Check sheet for the modelled part. Datum: model origin and axes. Units: mm. A direction names the side the tool comes from. Coordinates: 2 decimals unless noted, no trailing zeros. Write each loop counter-clockwise with the first axis right and the second up, starting at its lowest first coordinate (ties: lowest second). Pieces come first, ordered by that corner, then holes. Notation, with made-up numbers: M -25.75,-21 L 8.25,-21 A24 ccw 8.25,1 Z; hole C 26,6.5 d4. An arc over 180 degrees is marked long. Answer as CSV lines item,"result". Start each with the question number.
Q1. Sectioned sample at D-D, the plane z = -7. Record the cut outline in (x, y).
Q2. Sectioned sample at A-A, the plane x = 8. Record the cut outline in (y, z).
Q3. Sectioned sample at B-B, the plane z = -50. Record the cut outline in (x, y), then the cut area to 3 significant figures.
Q4. Sectioned sample at C-C, the plane y = 24. Record the cut outline in (x, z).
Q5. Thickness scan on line 1 along Y through (x, z) = (93, -72.5); line 2 along Z through (x, y) = (-72.5, -3); line 3 along Z through (x, y) = (-60, 14.5). Record the ranges inside material, lowest first. Write a range as from..to.
Q6. Depth check by flat-ended pin: pin 1 Ø16.5 at (x, y) = (285, -3.5) entering from -Z; pin 2 Ø16.5 at (y, z) = (-9.5, -47) entering from +X; pin 3 Ø22 at (x, y) = (50.5, 21.5) entering from -Z. Enter the tip coordinate at first touch or a pass-through.
Q7. Access from +Z, -Z, +X, -X, +Y, -Y to the whole of each face (thin tool, end or side, straight path). Record for faces 1 (the flat face through (13, 12.5, -63)), 2 (the flat face through (255, -7, -43)), 3 (the flat face through (-265, -7, -17.5)).
from build123d import *

# Parameters (mm, degrees)
SKETCH053_W     = 610
SKETCH053_H     = 165
PAD005_DEPTH    = 65
SKETCH054_W     = 60
SKETCH054_H     = 32
SKETCH054_W_2   = 70
SKETCH054_H_2   = 18
POCKET047_DEPTH = 165.001
SKETCH055_W     = 80
SKETCH055_H     = 32
SKETCH055_W_2   = 90
SKETCH055_H_2   = 18
POCKET048_DEPTH = 165.001
SKETCH056_W     = 50
SKETCH056_H     = 65
POCKET049_DEPTH = 65.001
SKETCH057_W     = 65
SKETCH057_H     = 65
POCKET050_DEPTH = 65.001
SKETCH059_W     = 610
SKETCH059_H     = 32
POCKET052_DEPTH = 10
SKETCH060_W     = 20
SKETCH060_H     = 25
POCKET053_DEPTH = 610.001
SKETCH061_W     = 50
SKETCH061_H     = 15
POCKET054_DEPTH = 610.001
SKETCH062_W     = 15
SKETCH062_H     = 65
POCKET055_DEPTH = 165.001
SKETCH063_W     = 10
SKETCH063_H     = 32.5
POCKET056_DEPTH = 165.001


with BuildPart() as part:
    # Sketch053 (on DatumPlane) → Pad005 (new body)
    with BuildSketch(Plane.XZ.offset(32.5)):
        Rectangle(SKETCH053_W, SKETCH053_H)
    extrude(amount=-PAD005_DEPTH)

    # Sketch054 (on DatumPlane) → Pocket047 (cut, through all)
    with BuildSketch(Plane.XY.offset(82.5)):
        with Locations((275, 16.5)):
            Rectangle(SKETCH054_W, SKETCH054_H)
        with Locations((270, -23.5)):
            Rectangle(SKETCH054_W_2, SKETCH054_H_2)
    extrude(amount=-POCKET047_DEPTH, mode=Mode.SUBTRACT)

    # Sketch055 (on DatumPlane) → Pocket048 (cut, through all)
    with BuildSketch(Plane.XY.offset(82.5)):
        with Locations((-265, 16.5)):
            Rectangle(SKETCH055_W, SKETCH055_H)
        with Locations((-260, -23.5)):
            Rectangle(SKETCH055_W_2, SKETCH055_H_2)
    extrude(amount=-POCKET048_DEPTH, mode=Mode.SUBTRACT)

    # Sketch056 (on DatumPlane) → Pocket049 (cut, through all)
    with BuildSketch(Plane.XZ.offset(32.5)):
        with Locations((280, -50)):
            Rectangle(SKETCH056_W, SKETCH056_H)
    extrude(amount=-POCKET049_DEPTH, mode=Mode.SUBTRACT)

    # Sketch057 (on DatumPlane) → Pocket050 (cut, through all)
    with BuildSketch(Plane.XZ.offset(32.5)):
        with Locations((-272.5, -50)):
            Rectangle(SKETCH057_W, SKETCH057_H)
    extrude(amount=-POCKET050_DEPTH, mode=Mode.SUBTRACT)

    # Sketch059 (on DatumPlane) → Pocket052 (cut)
    with BuildSketch(Plane.XY.offset(82.5)):
        with Locations((0, 16.5)):
            Rectangle(SKETCH059_W, SKETCH059_H)
    extrude(amount=-POCKET052_DEPTH, mode=Mode.SUBTRACT)

    # Sketch060 (on DatumPlane) → Pocket053 (cut, through all)
    with BuildSketch(Plane.YZ.offset(305)):
        with Locations((22.5, -70)):
            Rectangle(SKETCH060_W, SKETCH060_H)
    extrude(amount=-POCKET053_DEPTH, mode=Mode.SUBTRACT)

    # Sketch061 (on DatumPlane) → Pocket054 (cut, through all)
    with BuildSketch(Plane.YZ.offset(305)):
        with Locations((7.5, -75)):
            Rectangle(SKETCH061_W, SKETCH061_H)
    extrude(amount=-POCKET054_DEPTH, mode=Mode.SUBTRACT)

    # Sketch062 (on DatumPlane) → Pocket055 (cut, through all)
    with BuildSketch(Plane.XY.offset(82.5)):
        with Locations((-297.5, 0)):
            Rectangle(SKETCH062_W, SKETCH062_H)
    extrude(amount=-POCKET055_DEPTH, mode=Mode.SUBTRACT)

    # Sketch063 (on DatumPlane) → Pocket056 (cut, through all)
    with BuildSketch(Plane.XY.offset(82.5)):
        with Locations((300, -16.25)):
            Rectangle(SKETCH063_W, SKETCH063_H)
    extrude(amount=-POCKET056_DEPTH, mode=Mode.SUBTRACT)


solid = part.part
Output:
1,outline,"M -290,-14.5 L -215,-14.5 L -215,-32.5 L 235,-32.5 L 235,-14.5 L 295,-14.5 L 295,0 L 305,0 L 305,0.5 L 245,0.5 L 245,32.5 L -225,32.5 L -225,0.5 L -290,0.5 Z"
2,outline,"M -32.5,-82.5 L -17.5,-82.5 L -17.5,-67.5 L 12.5,-67.5 L 12.5,-57.5 L 32.5,-57.5 L 32.5,72.5 L 0.5,72.5 L 0.5,82.5 L -32.5,82.5 Z"
3,outline,"M -240,-14.5 L -215,-14.5 L -215,-32.5 L 235,-32.5 L 235,-14.5 L 255,-14.5 L 255,0.5 L 245,0.5 L 245,32.5 L -225,32.5 L -225,0.5 L -240,0.5 Z"
3,area,"30,600 mm^2"
4,outline,"M -225,-57.5 L 245,-57.5 L 245,72.5 L -225,72.5 Z"
5,line 1,"y = -32.5..-17.5"
5,line 2,"z = -67.5..82.5"
5,line 3,"z = -57.5..72.5"
6,pin 1,"stops at z = -17.5"
6,pin 2,"stops at x = 255"
6,pin 3,"stops at z = -67.5"
7,face 1,"-Z, +X, -X, +Y"
7,face 2,"-Z, +X, +Y, -Y"
7,face 3,"-Z, -X, +Y, -Y"
